```python
from build123d import *

# Parameters (mm, degrees)
F0_W     = 609.6
F0_H     = 812.8
F1_DEPTH = 914.4
F4_DEPTH = 609.601
F3_W     = 457.2
F3_H     = 330.2
F5_DEPTH = 736.6
F6_DEPTH = 50.8


with BuildPart() as f1:
    # F0 (on Top) → F1 (new body)
    with BuildSketch(Plane.XY):
        Rectangle(F0_W, F0_H)
    extrude(amount=F1_DEPTH)

    # F2 (on face) → F4 (cut, through all)
    with BuildSketch(Plane.YZ.offset(304.8)):
        with BuildLine():
            Line((330.2, 56.8088516593), (330.2, 304.8))
            ThreePointArc((330.2, 304.8), (0, 381), (-330.2, 304.8))
            Line((-330.2, 304.8), (-330.2, 56.8088516593))
            Line((-330.2, 56.8088516593), (330.2, 56.8088516593))
        make_face()
    extrude(amount=-F4_DEPTH, mode=Mode.SUBTRACT)

    # F3 (on face) → F5 (cut)
    with BuildSketch(Plane.XZ.offset(406.4)):
        with Locations((0, 698.5)):
            Rectangle(F3_W, F3_H)
    extrude(amount=-F5_DEPTH, mode=Mode.SUBTRACT)

    # F6 (cut): a face of the model
    f6_faces = [f1.faces().sort_by_distance(p)[0] for p in [
        (0, 0, 914.4),
    ]]
    extrude(f6_faces, amount=-F6_DEPTH, mode=Mode.SUBTRACT)


solid = f1.part
```
Part model, mm, in its own coordinate system. A direction names the side the tool comes from. Give positions to 0.01 mm unless a question says otherwise; leave off trailing zeros. Order: outer loops, then holes, each group sorted by start corner. A loop starts at its lowest first (then second) coordinate and runs counter-clockwise, first axis right, second up. Notation, with made-up numbers: M -1.75,-1 L 9.25,-1 A34 cw 9.25,34 Z; hole C -38.5,20 d7. An arc over 180 degrees is marked long. Use a Markdown table: item, result. Add a question column.
(1) Probe line 1 along X through (y, z) = (22.5, 620.5); line 2 along Y through (x, z) = (163.5, 73.5); line 3 along Y through (x, z) = (-124, 612). List the from-to ranges inside material, lowest first. Write a range as [from, to].
(2) Mould opens along Y. For faces 4 (the face through (-4, 406.4, 426)), 5 (the face through (4, -330.2, 183)), 6 (the face through (228.6, -43, 696)) say: +Y half, -Y half, draft (parallel to the pull), parting line (faces both ways), or undercut.
(3) Saw through at A-A, the plane x = -246.5. Give the cut face in (y, z), and give its area (3 significant figures).
(4) Drop a flat-ended pin along its axis: P1, Ø2, axis at x = -199.5, y = 300, coming from the +Z side. Give the stop position or say it passes through.
(5) 3-axis set-ups, long thin cutter, end or side, ignore diameter. For faces 1 (the face through (4.267, 4.785, 380.985)), 2 (the face through (-3, -43, 533.4)), 3 (the face through (-24, 333, 863.6)): which of +Z, -Z, +X, -X, +Y, -Y reach the whole face in a straight line?
(6) Saw through at D-D, the plane x = 1.5. Give the cut face in (y, z), and give its area (3 significant figures).
(7) Saw through at B-B, the plane y = 290. Give the cut face in (x, z).
(8) Saw through at C-C, the plane z = 126. Give the cut face in (x, y).
Answer key:
| question | item | result |
|---|---|---|
| 1 | line 1 | [-304.8, -228.6], [228.6, 304.8] |
| 1 | line 2 | [-406.4, -330.2], [330.2, 406.4] |
| 1 | line 3 | [330.2, 406.4] |
| 2 | face 4 | +Y half |
| 2 | face 5 | undercut |
| 2 | face 6 | draft |
| 3 | outline | M -406.4,0 L 406.4,0 L 406.4,863.6 L -406.4,863.6 Z; hole M -330.2,56.81 L 330.2,56.81 L 330.2,304.8 A753.53 ccw -330.2,304.8 Z |
| 3 | area | 504,000 mm^2 |
| 4 | P1 | z = 533.4 |
| 5 | face 1 | +X, -X |
| 5 | face 2 | +Z, -Y |
| 5 | face 3 | +Z, +X, -X, +Y, -Y |
| 6 | outline | M -406.4,0 L 406.4,0 L 406.4,863.6 L 330.2,863.6 L 330.2,533.4 L -406.4,533.4 Z; hole M -330.2,56.81 L 330.2,56.81 L 330.2,304.8 A753.53 ccw -330.2,304.8 Z |
| 6 | area | 261,000 mm^2 |
| 7 | outline | M -304.8,0 L 304.8,0 L 304.8,56.81 L -304.8,56.81 Z; M -304.8,322.96 L 304.8,322.96 L 304.8,863.6 L 228.6,863.6 L 228.6,533.4 L -228.6,533.4 L -228.6,863.6 L -304.8,863.6 Z |
| 8 | outline | M -304.8,-406.4 L 304.8,-406.4 L 304.8,-330.2 L -304.8,-330.2 Z; M -304.8,330.2 L 304.8,330.2 L 304.8,406.4 L -304.8,406.4 Z |
